from build123d import *

# Parameters (mm, degrees)
SKETCH1_R           = 2.25
BOSS_EXTRUDE1_DEPTH = 5
SKETCH2_R           = 2.25
CUT_EXTRUDE2_DEPTH  = 43.426406871
SKETCH4_W           = 11
SKETCH4_H           = 8
CUT_EXTRUDE5_DEPTH  = 42.533119315
SKETCH5_W           = 16
SKETCH5_H           = 5
CUT_EXTRUDE6_DEPTH  = 42.533119315


with BuildPart() as part:
    # Sketch1 → Boss-Extrude1 (new, symmetric)
    with BuildSketch(Plane.XY):
        with BuildLine():
            Line((0, 5), (40, 5))
            Line((40, 5), (40, -5))
            Line((40, -5), (0, -5))
            ThreePointArc((0, -5), (-5, 0), (0, 5))
        make_face()
        Circle(SKETCH1_R, mode=Mode.SUBTRACT)
    extrude(amount=BOSS_EXTRUDE1_DEPTH, both=True)

    # Sketch2 → Cut-Extrude2 (cut, through all)
    with BuildSketch(Plane(origin=(0, -5, 5), x_dir=(1, 0, 0), z_dir=(0, 0, -1))):
        with Locations(Location((22, -5, 0), (0, 0, 180))):
            Circle(SKETCH2_R)
    extrude(amount=CUT_EXTRUDE2_DEPTH, mode=Mode.SUBTRACT)

    # Sketch4 → Cut-Extrude5 (cut, through all)
    with BuildSketch(Plane(origin=(0, 0, 5), x_dir=(-1, 0, 0), z_dir=(0, 0, -1))):
        with Locations((-33.5, 0)):
            Rectangle(SKETCH4_W, SKETCH4_H)
    extrude(amount=CUT_EXTRUDE5_DEPTH, mode=Mode.SUBTRACT)

    # Sketch5 → Cut-Extrude6 (cut, through all)
    with BuildSketch(Plane.XZ.offset(5)):
        with Locations((3, 0)):
            Rectangle(SKETCH5_W, SKETCH5_H)
    extrude(amount=-CUT_EXTRUDE6_DEPTH, mode=Mode.SUBTRACT)


solid = part.part
Design review of the part built by this model. Coordinates are the model's own, in mm. A direction names the side the tool comes from. Give positions to 0.01 mm unless a question says otherwise; leave off trailing zeros. Loops run counter-clockwise (first coordinate to the right, second up) from the corner with the lowest first, then second, coordinate; pieces in that order, holes last. Notation, with made-up numbers: M 4.25,1 L 21.25,1 A24 cw 21.25,25 Z; hole C 61,13.5 d2. An arc over 180 degrees is marked long. Write item = value, one per line.
Q1. We need section B-B (y = 0). Give the boundary of the cut face in (x, z), plus the area to 4 significant figures.
Output values:
outline = M -5,-5 L -2.25,-5 L -2.25,-2.5 L -5,-2.5 Z; M -5,2.5 L -2.25,2.5 L -2.25,5 L -5,5 Z; M 2.25,-5 L 19.75,-5 L 19.75,5 L 2.25,5 L 2.25,2.5 L 11,2.5 L 11,-2.5 L 2.25,-2.5 Z; M 24.25,-5 L 28,-5 L 28,5 L 24.25,5 Z; M 39,-5 L 40,-5 L 40,5 L 39,5 Z
area = 192.5 mm^2
Q2. Draft analysis for pull direction Y (two halves, no side actions). For faces 1 (the flat face through (39, 0, 0)), 2 (the flat face through (3, 0, -2.5)), 3 (the flat face through (20, -5, 0)), 4 (the flat face through (34, -4, 0)), state which applies: +Y half, -Y half, draft (parallel to the pull), parting line (faces both ways), or undercut.
Output values:
face_1 = undercut
face_2 = draft
face_3 = -Y half
face_4 = undercut
Q3. Insertion check: pin 1 (1.5 mm diameter, centred on x = 32, y = 3, fed in from +Z); pin 2 (1.5 mm diameter, centred on y = 1.5, z = 0.5, fed in from -X). Each pin has a flat end and moves straight along its axis. Give the tip position at first contact, or say it passes through.
Output values:
pin_1 = through
pin_2 = 11
Q4. To check wall thickness, follow line 1 (X direction, y = 0, z = -3.95); line 2 (X direction, y = 0, z = 0.5); line 3 (Z direction, x = 5, y = 2). State the ranges of each line that lie inside material, in increasing order. Write a range as [from, to].
Output values:
line_1 = [-5, -2.25], [2.25, 19.75], [24.25, 28], [39, 40]
line_2 = [11, 19.75], [24.25, 28], [39, 40]
line_3 = [-5, -2.5], [2.5, 5]
Q5. We need section A-A (x = 4). Give the boundary of the cut face in (y, z).
Output values:
outline = M -5,-5 L 5,-5 L 5,-2.5 L -5,-2.5 Z; M -5,2.5 L 5,2.5 L 5,5 L -5,5 Z
Q6. We need section C-C (z = -2). Give the boundary of the cut face in (x, y), plus the area to 3 significant figures.
Output values:
outline = M 11,-5 L 40,-5 L 40,5 L 11,5 Z; hole C 22,0 d4.5; hole M 28,-4 L 39,-4 L 39,4 L 28,4 Z
area = 186 mm^2
Q7. For faces 5 (the flat face through (34, 4, 0)), 6 (the flat face through (24, 5, 0)), 7 (the flat face through (3, 0, 2.5)), list the 3-axis set-ups (+Z, -Z, +X, -X, +Y, -Y) from which the entire face can be reached by the end or side of a thin tool; tool diameter is ignored.
Output values:
face_5 = +Z, -Z
face_6 = +Z, -Z, +X, -X, +Y
face_7 = -X, +Y, -Y
Q8. We need section D-D (x = 22). Give the boundary of the cut face in (y, z), plus the area to 3 significant figures.
Output values:
outline = M -5,-5 L -2.25,-5 L -2.25,5 L -5,5 Z; M 2.25,-5 L 5,-5 L 5,5 L 2.25,5 Z
area = 55.0 mm^2
